Model file for the job. Use its own axes, mm. A direction names the side the tool comes from. Coordinates: 2 decimals unless noted, no trailing zeros. Write each loop counter-clockwise with the first axis right and the second up, starting at its lowest first coordinate (ties: lowest second). Pieces come first, ordered by that corner, then holes. Notation, with made-up numbers: M 0.5,0 L 50.5,0 A12 cw 50.5,20 Z; hole C 68.5,8.5 d10. An arc over 180 degrees is marked long. Put each result on its own line as item: value. Start each with the question number.
Q1. Cut at C-C (y = 24.5). Give the number of separate pieces and of enclosed holes in the cut face, then the cut area to 3 significant figures.
Q2. Pull direction Z, two halves, no side cores. Call faces 1 (the flat face through (-1.4, 26.415, 2.6)), 2 (the flat face through (28.708, 18, 24)), 3 (the cylindrical face through (56.181, 21.598, -34.203)), 4 (the flat face through (-3.642, 22, -16)): pulls with the +Z half, pulls with the -Z half, needs draft (parallel to the pull), parting line crosses it, or undercut.
Q3. Drop flat-ended pins along their axis: pin 1 (0.8 mm diameter, centred on y = 18, z = 12, fed in from -X); pin 2 (2 mm diameter, centred on x = 5.5, z = -9.5, fed in from +Y); pin 3 (0.8 mm diameter, centred on x = -2.5, z = 13, fed in from -Y); pin 4 (1.3 mm diameter, centred on x = -1.27, z = -28.97, fed in from +Y). Give the stop position or say it passes through.
Q4. Cut at B-B (x = 1). Write the cut outline in (y, z), then the cut area to 3 significant figures.
Q5. Which spindle directions (+Z, -Z, +X, -X, +Y, -Y) get a long thin tool onto all of the face, cutting with end or side? Do faces 5 (the flat face through (36, 21.415, 35)), 6 (the flat face through (-3.142, 24, 7)), 7 (the flat face through (4.749, 18, 26)). Say none if no direction does.
Q6. Cut at A-A (x = 22). Write the cut outline in (y, z).
Q7. Cut at D-D (z = -17.5). Write the cut outline in (x, y).
Q8. Drill centre lines: line 1 along Z through (x, y) = (39, 20.5); line 2 along Z through (x, y) = (22.5, 17.5); line 3 along X through (y, z) = (23, 17). Where is each one in solid material? Low to high.
```python
from build123d import *

# Parameters (mm, degrees)
SKETCH2_W              = 64
SKETCH2_H              = 75.2942
BASE_DEPTH             = 1.5
SKETCH6_W              = 64
SKETCH6_H              = 75.2942
SKETCH6_W_2            = 57
SKETCH6_H_2            = 68.2942
OUTSIDE_WALLS_DEPTH    = 8
SKETCH3_W              = 44.5
SKETCH3_H              = 2.5
SKETCH3_W_2            = 37.65
DIVIDER_WALLS_DEPTH    = 3
USB_START              = 0.160298289
USB_HOLE_DEPTH         = 13.899833209
SKETCH10_W             = 3.5
SKETCH10_H             = 3.5
BATT_MT3608_STOP_DEPTH = 3
TP4056_START           = 18.414945084
TP4056_STOP_OUTLINE_W  = 2.5
TP4056_STOP_OUTLINE_H  = 3.0942
TP4056_STOP_DEPTH      = 3
WIRE_START             = 20.416440404
WIRE_HOLES_OUTLINE_W   = 1.5
WIRE_HOLES_OUTLINE_H   = 6.588
WIRE_HOLES_DEPTH       = 8.3622
WIRE_START_2           = -3.642059596
WIRE_HOLES_2_OUTLINE_W = 1.5
WIRE_HOLES_2_OUTLINE_H = 13
WIRE_HOLES_2_DEPTH     = 8.390953786
WIRE_START_3           = 28.707940404
WIRE_HOLES_3_OUTLINE_W = 1.5
WIRE_HOLES_3_OUTLINE_H = 4
WIRE_HOLES_3_DEPTH     = 11
WIRE_START_4           = 4.74889419
WIRE_HOLES_4_OUTLINE_W = 1.5
WIRE_HOLES_4_OUTLINE_H = 4.98430333
WIRE_HOLES_4_DEPTH     = 8.028885191
USB_HOOD_DEPTH         = 2.5
USB_BACKING_DEPTH      = 2
SKETCH19_W             = 2.5
SKETCH19_H             = 18.0942
CUT_EXTRUDE2_DEPTH     = 1.5
SKETCH16_R             = 1.125
SCREW_HOLES_DEPTH      = 6
FILLET1_R              = 2.25
BOSS_EXTRUDE3_START    = 6.25
SKETCH17_W             = 3.5
SKETCH17_H             = 6
SKETCH17_R             = 1.125
SKETCH17_H_2           = 5
BOSS_EXTRUDE3_DEPTH    = 6.25
SKETCH18_R             = 1.125
CUT_EXTRUDE1_DEPTH     = 1.5


# Read off the part's stored shape, not the designer's step: USB Hole, TP4056 Stop, Wire Holes
with BuildPart() as part:
    # Sketch2 → Base (new body)
    with BuildSketch(Plane.XZ.offset(-18.414945084)):
        with Locations((24.857940404, 2.802763775)):
            Rectangle(SKETCH2_W, SKETCH2_H)
    extrude(amount=BASE_DEPTH)

    # Sketch6 → Outside Walls (add)
    with BuildSketch(Plane(origin=(0, 18.414945084, 0), x_dir=(1, 0, 0), z_dir=(0, 1, 0))):
        with Locations((24.857940404, -2.802763775)):
            Rectangle(SKETCH6_W, SKETCH6_H)
        with Locations((24.857940404, -2.802763775)):
            Rectangle(SKETCH6_W_2, SKETCH6_H_2, mode=Mode.SUBTRACT)
    extrude(amount=OUTSIDE_WALLS_DEPTH)

    # Sketch3 → Divider Walls (add)
    with BuildSketch(Plane(origin=(0, 18.414945084, 0), x_dir=(1, 0, 0), z_dir=(0, 1, 0))):
        with Locations((18.607940404, 3.094336225)):
            Rectangle(SKETCH3_W, SKETCH3_H)
        with Locations((15.182940404, -17.499863775)):
            Rectangle(SKETCH3_W_2, SKETCH3_H)
    extrude(amount=DIVIDER_WALLS_DEPTH)

    # USB Hole outline → USB Hole (cut)
    with BuildSketch(Plane.XY.offset(USB_START)):
        Polygon((-3.142059596, 16.914945084), (-3.142059596, 18.414945084), (-3.642059596, 18.414945084), (-3.642059596, 25.689688961), (-7.142059596, 25.689688961), (-7.142059596, 16.914945084), align=None)
    extrude(amount=USB_HOLE_DEPTH, mode=Mode.SUBTRACT)

    # Sketch10 → Batt & MT3608 Stop (add)
    with BuildSketch(Plane(origin=(0, 18.414945084, 0), x_dir=(1, 0, 0), z_dir=(0, 1, 0))):
        Polygon((44.857940404, 1.844336225), (40.857940404, 1.844336225), (40.857940404, 4.344336225), (41.357940404, 4.344336225), (41.357940404, 11.844336225), (44.857940404, 11.844336225), align=None)
        Polygon((34.507940404, -18.749863775), (34.007940404, -18.749863775), (34.007940404, -16.249863775), (38.007940404, -16.249863775), (38.007940404, -22.249863775), (34.507940404, -22.249863775), align=None)
        with Locations((36.257940404, -35.199863775)):
            Rectangle(SKETCH10_W, SKETCH10_H)
    extrude(amount=BATT_MT3608_STOP_DEPTH)

    # TP4056 Stop outline → TP4056 Stop (add)
    with BuildSketch(Plane(origin=(0, 0, 0), x_dir=(1, 0, 0), z_dir=(0, 1, 0)).offset(TP4056_START)):
        with Locations((25.107940404, -7.202763775)):
            Rectangle(TP4056_STOP_OUTLINE_W, TP4056_STOP_OUTLINE_H)
    extrude(amount=TP4056_STOP_DEPTH)

    # Wire Holes outline → Wire Holes (cut)
    with BuildSketch(Plane.YZ.offset(WIRE_START)):
        with Locations((17.664945084, 12.574863775)):
            Rectangle(WIRE_HOLES_OUTLINE_W, WIRE_HOLES_OUTLINE_H)
        with Locations((17.664945084, 1.830663775)):
            Rectangle(WIRE_HOLES_OUTLINE_W, WIRE_HOLES_OUTLINE_H)
    extrude(amount=WIRE_HOLES_DEPTH, mode=Mode.SUBTRACT)

    # Wire Holes 2 outline → Wire Holes 2 (cut)
    with BuildSketch(Plane.YZ.offset(WIRE_START_2)):
        with Locations((17.664945084, 27.849863775)):
            Rectangle(WIRE_HOLES_2_OUTLINE_W, WIRE_HOLES_2_OUTLINE_H)
    extrude(amount=WIRE_HOLES_2_DEPTH, mode=Mode.SUBTRACT)

    # Wire Holes 3 outline → Wire Holes 3 (cut)
    with BuildSketch(Plane.YZ.offset(WIRE_START_3)):
        with Locations((17.664945084, 24.249863775)):
            Rectangle(WIRE_HOLES_3_OUTLINE_W, WIRE_HOLES_3_OUTLINE_H)
        with Locations((17.664945084, 31.449863775)):
            Rectangle(WIRE_HOLES_3_OUTLINE_W, WIRE_HOLES_3_OUTLINE_H)
    extrude(amount=WIRE_HOLES_3_DEPTH, mode=Mode.SUBTRACT)

    # Wire Holes 4 outline → Wire Holes 4 (cut)
    with BuildSketch(Plane.YZ.offset(WIRE_START_4)):
        with Locations((17.664945084, 32.272120623)):
            Rectangle(WIRE_HOLES_4_OUTLINE_W, WIRE_HOLES_4_OUTLINE_H)
    extrude(amount=WIRE_HOLES_4_DEPTH, mode=Mode.SUBTRACT)

    # Sketch14 → USB Hood (add)
    with BuildSketch(Plane(origin=(-3.642059596, 0, 0), x_dir=(0, 0, -1), z_dir=(1, 0, 0))):
        Polygon((-14.060131498, 19.989745084), (-14.060131498, 25.689688961), (-0.160298289, 25.689688961), (-0.160298289, 19.989745084), (1.844336225, 19.989745084), (1.844336225, 26.414945084), (-16.249863775, 26.414945084), (-16.249863775, 19.989745084), align=None)
    extrude(amount=USB_HOOD_DEPTH)

    # Sketch15 → USB Backing (add)
    with BuildSketch(Plane(origin=(-1.142059596, 0, 0), x_dir=(0, 0, -1), z_dir=(1, 0, 0))):
        Polygon((-2.681738903, 22.989735785), (-2.681738903, 20.961450556), (-3.59783083, 19.989745084), (-0.160298289, 19.989745084), (-0.160298289, 25.689688961), (-14.060131498, 25.689688961), (-14.060131498, 19.989745084), (-10.622685302, 19.989745084), (-11.538656584, 20.961320912), (-11.538656584, 22.989735785), align=None)
    extrude(amount=-USB_BACKING_DEPTH)

    # Sketch19 → Cut-Extrude2 (cut)
    with BuildSketch(Plane(origin=(0, 18.414945084, 0), x_dir=(1, 0, 0), z_dir=(0, 1, 0))):
        with Locations((-2.392059596, -7.202763775)):
            Rectangle(SKETCH19_W, SKETCH19_H)
    extrude(amount=-CUT_EXTRUDE2_DEPTH, mode=Mode.SUBTRACT)

    # Sketch16 → Screw Holes (cut)
    with BuildSketch(Plane(origin=(0, 26.414945084, 0), x_dir=(1, 0, 0), z_dir=(0, 1, 0))):
        with Locations(Location((-5.091807064, 32.794083694, 0), (0, 0, 180))):
            Circle(SKETCH16_R)
        with Locations((54.807687872, 32.794083694)):
            Circle(SKETCH16_R)
        with Locations((-5.091807064, -38.399611243)):
            Circle(SKETCH16_R)
        with Locations(Location((54.807687872, -38.399611243, 0), (0, 0, 180))):
            Circle(SKETCH16_R)
        with Locations(Location((43.107940404, 10.094336225, 0), (0, 0, 180))):
            Circle(SKETCH16_R)
        with Locations(Location((36.257940404, -20.199611243, 0), (0, 0, 180))):
            Circle(SKETCH16_R)
    extrude(amount=-SCREW_HOLES_DEPTH, mode=Mode.SUBTRACT)

    # Fillet1
    fillet1_edges = [part.edges().sort_by_distance(p)[0] for p in [
        (-7.142059596, 21.664945084, 40.449863775),
        (-7.142059596, 21.664945084, -34.844336225),
        (56.857940404, 21.664945084, -34.844336225),
        (56.857940404, 21.664945084, 40.449863775),
    ]]
    fillet(fillet1_edges, radius=FILLET1_R)

    # Sketch17 → Boss-Extrude3 (add)
    # profile 1 of 2: a face of its own
    with BuildSketch(Plane(origin=(0, 21.414945084, 0), x_dir=(1, 0, 0), z_dir=(0, 1, 0)).offset(BOSS_EXTRUDE3_START)):
        with Locations((36.257940404, -19.249863775)):
            Rectangle(SKETCH17_W, SKETCH17_H)
        with Locations(Location((36.257940404, -20.199611243, 0), (0, 0, 180))):
            Circle(SKETCH17_R, mode=Mode.SUBTRACT)
    # profile 2 of 2: a face of its own
    with BuildSketch(Plane(origin=(0, 21.414945084, 0), x_dir=(1, 0, 0), z_dir=(0, 1, 0)).offset(BOSS_EXTRUDE3_START)):
        with Locations((43.107940404, 9.344336225)):
            Rectangle(SKETCH17_W, SKETCH17_H_2)
        with Locations(Location((43.107940404, 10.094336225, 0), (0, 0, 180))):
            Circle(SKETCH17_R, mode=Mode.SUBTRACT)
    extrude(amount=-BOSS_EXTRUDE3_DEPTH)

    # Sketch18 → Cut-Extrude1 (cut)
    with BuildSketch(Plane.XZ.offset(-16.914945084)):
        with Locations((50.982940404, 34.574863775)):
            Circle(SKETCH18_R)
        with Locations((50.982940404, 2.802763775)):
            Circle(SKETCH18_R)
        with Locations((50.982940404, -28.969336225)):
            Circle(SKETCH18_R)
        with Locations((-1.267059596, -28.969336225)):
            Circle(SKETCH18_R)
        with Locations((7.12389419, 21.124863775)):
            Circle(SKETCH18_R)
    extrude(amount=-CUT_EXTRUDE1_DEPTH, mode=Mode.SUBTRACT)


solid = part.part
```
Computed values:
1. separate pieces: 3
1. enclosed holes: 7
1. area: 926 mm2
2. face 1: needs draft
2. face 2: undercut
2. face 3: pulls with the -Z half
2. face 4: undercut
3. pin 1: x = -1.14
3. pin 2: y = 18.41
3. pin 3: y = 19.99
3. pin 4: through
4. outline: M 16.91,-34.84 L 26.41,-34.84 L 26.41,-31.34 L 18.41,-31.34 L 18.41,-4.34 L 21.41,-4.34 L 21.41,-1.84 L 18.41,-1.84 L 18.41,16.25 L 21.41,16.25 L 21.41,18.75 L 18.41,18.75 L 18.41,21.35 L 16.91,21.35 Z; M 16.91,34.35 L 18.41,34.35 L 18.41,36.95 L 26.41,36.95 L 26.41,40.45 L 16.91,40.45 Z
4. area: 164 mm2
5. face 5: +Y
5. face 6: -X, -Y
5. face 7: +Y, -Y
6. outline: M 16.91,-34.84 L 26.41,-34.84 L 26.41,-31.34 L 18.41,-31.34 L 18.41,-4.34 L 21.41,-4.34 L 21.41,-1.84 L 18.41,-1.84 L 18.41,-1.46 L 16.91,-1.46 Z; M 16.91,5.12 L 18.41,5.12 L 18.41,9.28 L 16.91,9.28 Z; M 16.91,15.87 L 18.41,15.87 L 18.41,16.25 L 21.41,16.25 L 21.41,18.75 L 18.41,18.75 L 18.41,36.95 L 26.41,36.95 L 26.41,40.45 L 16.91,40.45 Z
7. outline: M -7.14,16.91 L 56.86,16.91 L 56.86,26.41 L 53.36,26.41 L 53.36,18.41 L -3.64,18.41 L -3.64,26.41 L -7.14,26.41 Z
8. line 1: -34.84 to -31.34, -4.34 to -1.84, 36.95 to 40.45
8. line 2: -34.84 to -1.46, 5.12 to 9.28, 15.87 to 40.45
8. line 3: -7.14 to -3.64, 34.51 to 38.01, 53.36 to 56.86
